from build123d import *

# Parameters (mm, degrees)
BOSS_EXTRUDE1_DEPTH = 15
SKETCH4_R           = 7.5
CUT_EXTRUDE1_DEPTH  = 30.270292107


with BuildPart() as part:
    # Sketch3 → Boss-Extrude1 (new body)
    with BuildSketch(Plane(origin=(0, 0, 0), x_dir=(1, 0, 0), z_dir=(0, 1, 0))):
        Polygon((0, -19), (16.454482672, -9.5), (16.454482672, 9.5), (0, 19), (-16.454482672, 9.5), (-16.454482672, -9.5), align=None)
    extrude(amount=BOSS_EXTRUDE1_DEPTH)

    # Sketch4 → Cut-Extrude1 (cut, through all)
    with BuildSketch(Plane(origin=(0, 15, 0), x_dir=(1, 0, 0), z_dir=(0, 1, 0))):
        with Locations(Location((0, 0, 0), (0, 0, 270))):
            Circle(SKETCH4_R)
    extrude(amount=-CUT_EXTRUDE1_DEPTH, mode=Mode.SUBTRACT)

    # Sketch6 → Cut-Revolve1 (revolve, cut)
    with BuildSketch(Plane(origin=(0, 0, 0), x_dir=(0, 0, -1), z_dir=(1, 0, 0))):
        Polygon((16.222397812, 15.777602188), (21.222397812, 10.777602188), (21.222397812, 15.777602188), align=None)
    revolve(axis=Axis((0, 0, 0), (0, 1, 0)), mode=Mode.SUBTRACT)

    # Sketch8 → Cut-Revolve2 (revolve, cut)
    with BuildSketch(Plane(origin=(0, 0, 0), x_dir=(0, 0, -1), z_dir=(1, 0, 0))):
        Polygon((16.303352357, -0.696647643), (21.303352357, 4.303352357), (21.303352357, -0.696647643), align=None)
    revolve(axis=Axis((0, 0, 0), (0, 1, 0)), mode=Mode.SUBTRACT)


solid = part.part
For this review, take the finished solid that the model builds, in its own axes (mm). Round coordinates to 2 decimals unless told otherwise and drop trailing zeros. Write each loop counter-clockwise with the first axis right and the second up, starting at its lowest first coordinate (ties: lowest second). Pieces come first, ordered by that corner, then holes. Notation, with made-up numbers: (31.5, 14.5) - (83.5, 14.5) arc R24 ccw to (83.5, 32.5) - close; hole circle Ø1 at (-18.75, 16.25). An arc over 180 degrees is marked (long way). Write item = value, one per line. Start each with the question number.
1. Consider section B-B on y = 7.25. State the section outline as (x, z) points, plus the area to 3 significant figures.
2. Consider section D-D on z = -15.5. State the section outline as (x, y) points, plus the area to 3 significant figures.
3. Consider section C-C on x = 5. State the section outline as (y, z) points.
4. Consider section A-A on z = 0. State the section outline as (x, y) points, plus the area to 3 significant figures.
5. Wall thickness on L1, parallel to X at y = 9.75, z = 0; L2, parallel to X at y = 6, z = 1.5; L3, parallel to Z at x = -5, y = 11.5: over which ranges is each line inside the solid? List them lowest first.
6. For pin 1 Ø2 at (x, y) = (-5.5, 2) entering from -Z; pin 2 Ø5 at (x, y) = (-0.5, 3) entering from -Z; pin 3 Ø5 at (x, y) = (-5.5, 7.5) entering from -Z; pin 4 Ø3 at (x, y) = (8, 4.5) entering from -Z, all flat-tipped, find the tip position at first contact; note any pin that passes through.
7. Draft analysis for pull direction Z (two halves, no side actions). For faces 1 (the face through (0.33, 7.605, -7.493)), 2 (the face through (-8, 0, 0)), 3 (the face through (-8.342, 7.395, 14.183)), 4 (the face through (15.25, 14.43, -8.73)), state which applies: released by +Z, released by -Z, zero draft, split by the parting line, or undercut.
Evaluation:
q1.outline = (-16.45, -9.5) - (0, -19) - (16.45, -9.5) - (16.45, 9.5) - (0, 19) - (-16.45, 9.5) - close; hole circle Ø15 at (0, 0)
q1.area = 761 mm2
q2.outline = (-6.06, 0) - (6.06, 0) - (6.06, 15) - (-6.06, 15) - close
q2.area = 182 mm2
q3.outline = (0, -16.11) - (15, -16.11) - (15, -5.59) - (0, -5.59) - close; (0, 5.59) - (15, 5.59) - (15, 16.11) - (0, 16.11) - close
q4.outline = (-16.45, 0) - (-7.5, 0) - (-7.5, 15) - (-16.45, 15) - close; (7.5, 0) - (16.45, 0) - (16.45, 15) - (7.5, 15) - close
q4.area = 269 mm2
q5.L1 = -16.45 to -7.5, 7.5 to 16.45
q5.L2 = -16.45 to -7.35, 7.35 to 16.45
q5.L3 = -16.11 to -5.59, 5.59 to 16.11
q6.pin_1 = -16.4
q6.pin_2 = -19
q6.pin_3 = -17.27
q6.pin_4 = -15.25
q7.face_1 = undercut
q7.face_2 = zero draft
q7.face_3 = released by +Z
q7.face_4 = released by -Z
